from build123d import *

# Parameters (mm, degrees)
SKETCH1_R            = 5
BOSS_EXTRUDE1_DEPTH  = 21
CHAMFER1_SIZE        = 1
BOSS_EXTRUDE2_START  = 61.7
BOSS_EXTRUDE2_DEPTH  = 61.7
BOSS_EXTRUDE5_START  = 11.8
SKETCH3_R            = 5
BOSS_EXTRUDE5_DEPTH  = 11.8
SKETCH5_R            = 3.45
BOSS_EXTRUDE6_DEPTH  = 2.5
BOSS_EXTRUDE7_START  = 15
SKETCH6_R            = 5
BOSS_EXTRUDE7_DEPTH  = 15
BOSS_EXTRUDE8_DEPTH  = 1.5
BOSS_EXTRUDE10_START = 10.5
SKETCH9_R            = 5
BOSS_EXTRUDE10_DEPTH = 10.5
CHAMFER3_SIZE        = 1
CUT_EXTRUDE1_DEPTH   = 10.5
SKETCH11_R           = 1.5
CUT_EXTRUDE2_DEPTH   = 10.5


with BuildPart() as part:
    # Sketch1 → Boss-Extrude1 (new body)
    with BuildSketch(Plane(origin=(0, 0, 0), x_dir=(0, 0, -1), z_dir=(1, 0, 0))):
        with Locations(Location((0, 0, 0), (0, 0, 180))):
            Circle(SKETCH1_R)
    extrude(amount=BOSS_EXTRUDE1_DEPTH)

    # Chamfer1
    chamfer1_edges = [part.edges().sort_by_distance(p)[0] for p in [
        (21, 0, -5),
    ]]
    chamfer(chamfer1_edges, length=CHAMFER1_SIZE)

    # Sketch2 → Boss-Extrude2 (add)
    with BuildSketch(Plane.ZY.offset(BOSS_EXTRUDE2_START)):
        with BuildLine():
            Line((-3.535533906, 3.535533906), (3.535533906, -3.535533906))
            ThreePointArc((3.535533906, -3.535533906), (-3.535533906, -3.535533906), (-3.535533906, 3.535533906))
        make_face()
    extrude(amount=-BOSS_EXTRUDE2_DEPTH)

    # Sketch3 → Boss-Extrude5 (add)
    with BuildSketch(Plane.ZY.offset(61.7).offset(BOSS_EXTRUDE5_START)):
        Circle(SKETCH3_R)
    extrude(amount=-BOSS_EXTRUDE5_DEPTH)

    # Sketch5 → Boss-Extrude6 (add)
    with BuildSketch(Plane.ZY.offset(73.5)):
        Circle(SKETCH5_R)
    extrude(amount=BOSS_EXTRUDE6_DEPTH)

    # Sketch6 → Boss-Extrude7 (add)
    with BuildSketch(Plane.ZY.offset(76).offset(BOSS_EXTRUDE7_START)):
        Circle(SKETCH6_R)
    extrude(amount=-BOSS_EXTRUDE7_DEPTH)

    # Sketch7 → Boss-Extrude8 (add)
    with BuildSketch(Plane.ZY.offset(91)):
        with BuildLine():
            Line((-2.861817604, 2.5), (2.861817604, 2.5))
            ThreePointArc((2.861817604, 2.5), (3.8, 0), (2.861817604, -2.5))
            Line((2.861817604, -2.5), (-2.861817604, -2.5))
            ThreePointArc((-2.861817604, -2.5), (-3.8, 0), (-2.861817604, 2.5))
        make_face()
    extrude(amount=BOSS_EXTRUDE8_DEPTH)

    # Sketch9 → Boss-Extrude10 (add)
    with BuildSketch(Plane.ZY.offset(92.5).offset(BOSS_EXTRUDE10_START)):
        Circle(SKETCH9_R)
    extrude(amount=-BOSS_EXTRUDE10_DEPTH)

    # Chamfer3
    chamfer3_edges = [part.edges().sort_by_distance(p)[0] for p in [
        (-103, 0, -5),
    ]]
    chamfer(chamfer3_edges, length=CHAMFER3_SIZE)

    # Sketch10 → Cut-Extrude1 (cut)
    with BuildSketch(Plane.ZY.offset(103)):
        with BuildLine():
            Line((-4.330127019, 2.5), (4.330127019, 2.5))
            ThreePointArc((4.330127019, 2.5), (0, 5), (-4.330127019, 2.5))
        make_face()
        with BuildLine():
            Line((-4.330127019, -2.5), (4.330127019, -2.5))
            ThreePointArc((4.330127019, -2.5), (0, -5), (-4.330127019, -2.5))
        make_face()
    extrude(amount=-CUT_EXTRUDE1_DEPTH, mode=Mode.SUBTRACT)

    # Sketch11 → Cut-Extrude2 (cut)
    with BuildSketch(Plane(origin=(0, 0, 0), x_dir=(1, 0, 0), z_dir=(0, 0.7071067811865468, 0.7071067811865483))):
        with Locations(Location((-12.85, 0, 0), (0, 0, 270))):
            Circle(SKETCH11_R)
        with Locations(Location((-48.85, 0, 0), (0, 0, 270))):
            Circle(SKETCH11_R)
    extrude(amount=-CUT_EXTRUDE2_DEPTH, mode=Mode.SUBTRACT)


solid = part.part
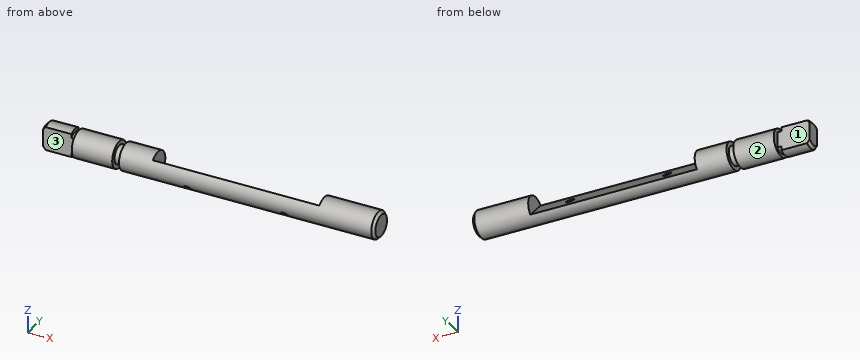
Work out the finished part from the listing and answer in its coordinate system (mm). Face numbers are marked on the shaded views. A direction names the side the tool comes from. Coordinates: 2 decimals unless noted, no trailing zeros. Write item = value, one per line.
1. For the marked faces 1, 2 and 3, determine the directions among +Z, -Z, +X, -X, +Y, -Y from which every point of the face is accessible in a straight line to the end or side of a thin tool.
Solution:
face_1 = +Z, -Z, -X, +Y
face_2 = +X, -X
face_3 = +Z, -Z, -X, -Y
2. Straight lines are drawn through the part: line 1 (X direction, y = -0.25, z = -0.25); line 2 (X direction, y = 0.5, z = 1.5); line 3 (X direction, y = -2.75, z = 3.75). For each, find the intervals that lie inside material, in ascending order. Write a range as from..to.
Solution:
line_1 = -103..-50.35, -47.35..-14.35, -11.35..21
line_2 = -103..-61.7, 0..21
line_3 = -91..-76, -73.5..-61.7, 0..20.35
3. Flat-ended cylindrical pins translate along their axes: pin 1 (1.1 mm diameter, centred on y = 0.5, z = -4, fed in from +X); pin 2 (1.5 mm diameter, centred on x = -8.5, z = -1.5, fed in from +Y); pin 3 (1.5 mm diameter, centred on x = -18, y = -1, fed in from +Z); pin 4 (1.5 mm diameter, centred on x = -55.5, y = 1.5, fed in from -Z). Find the tip coordinate at first contact, or state that the pin passes through.
Solution:
pin_1 = 21
pin_2 = 2.25
pin_3 = 1.75
pin_4 = -4.94
